Geometry: final body of the model. Coordinates: model frame, mm. Round coordinates to 2 decimals unless told otherwise and drop trailing zeros. Loops run counter-clockwise (first coordinate to the right, second up) from the corner with the lowest first, then second, coordinate; pieces in that order, holes last. Notation, with made-up numbers: (71.5, 49) - (103.5, 49) arc R16 ccw to (103.5, 54) - close; hole circle Ø3 at (-17.75, -30.5). An arc over 180 degrees is marked (long way). Write item = value, one per line. Start each with the question number.
Item 1: Line query: line 1 (X direction, y = 12.5, z = 10.25); line 2 (X direction, y = -12.5, z = 3.5); line 3 (Y direction, x = -6.5, z = 16). Output: solid intervals per line, ascending. Write a range as from..to.
Item 2: First-contact query: pin 1 (10 mm diameter, centred on y = -5, z = 22, fed in from -X); pin 2 (1.5 mm diameter, centred on x = 5.5, y = 12, fed in from +Z); pin 3 (4 mm diameter, centred on x = -9, y = -8, fed in from +Z). Flat tips, straight axial feed; report the tip coordinate or a pass-through.
Item 3: Section A-A (z = 18). Return loops of the section in (x, y).
from build123d import *

# Parameters (mm, degrees)
F2_W          = 32
F2_H          = 32
F3_DEPTH      = 20
F3_TAPER      = 38.6
F3_DEPTH_BACK = 8
F3_TAPER_BACK = 30


with BuildPart() as f3:
    # F2 (on plane+point) → F3 (new body, two sides)
    with BuildSketch(Plane.XY.offset(8)) as f3_sk:
        Rectangle(F2_W, F2_H)
    extrude(amount=F3_DEPTH, taper=F3_TAPER)
    extrude(f3_sk.sketch, amount=-F3_DEPTH_BACK, taper=F3_TAPER_BACK)


solid = f3.part
Taken from the geometry:
q1.line_1 = -14.2..14.2
q1.line_2 = -13.4..13.4
q1.line_3 = -9.61..9.61
q2.pin_1 = -8.82
q2.pin_2 = 13.95
q2.pin_3 = 19.05
q3.outline = (-8.02, -8.02) - (8.02, -8.02) - (8.02, 8.02) - (-8.02, 8.02) - close
